Autodesk Inventor part; units mm, degrees
ref_plane "YZ Plane" through (0, 0, 0) normal (1, 0, 0) x (0, 1, 0)
ref_plane "XZ Plane" through (0, 0, 0) normal (0, 1, 0) x (-1, 0, 0)
ref_plane "XY Plane" through (0, 0, 0) normal (0, 0, 1) x (1, 0, 0)
sketch "Sketch1" plane through (0, 0, 0) normal (0, 0, 1) x (1, 0, 0)
  circle A0 centre (8.9, 50.3645) radius 1.55 construction
  circle A1 centre (8.9, 50.3645) radius 3
  circle A2 centre (51.1, 50.3645) radius 1.55 construction
  circle A3 centre (51.1, 50.3645) radius 3
  circle A4 centre (60, 0) radius 1.55
  circle A5 centre (60, 0) radius 1.55
  circle A6 centre (0, 0) radius 1.55
  circle A7 centre (0, 0) radius 1.55
  circle A8 centre (54.13, 40.8) radius 1.5999
  circle A9 centre (5.87, 42.07) radius 1.5999
  circle A10 centre (38.89, -10) radius 1.5999
  circle A11 centre (54.13, 40.8) radius 1.55 construction
  circle A12 centre (5.87, 42.07) radius 1.55 construction
  circle A13 centre (38.89, -10) radius 1.55 construction
  line L0 (8.9, 55.3645) -> (3.9, 55.3645) construction
  circle A14 centre (30, 20) radius 22.5
  arc A15 (38.89, -5) -> (37.7654, -14.8719) centre (38.89, -10) ccw construction
  arc A16 (37.6448, -14.8425) -> (41.0305, -14.5186) centre (38.89, -10) ccw
  line L1 (8.9, 55.3645) -> (8.9, 50.3645) construction
  line L2 (51.1, 55.3645) -> (51.1, 50.3645) construction
  arc A17 (-1.2452, -4.8425) -> (-5, 0) centre (0, 0) ccw construction
  arc A18 (65, 0) -> (64.9237, 0.8701) centre (60, 0) ccw
  line L3 (-1.2452, -4.8425) -> (37.6448, -14.8425)
  line L4 (41.0305, -14.5186) -> (62.1405, -4.5186)
  arc A19 (-4.9237, 0.8701) -> (-1.2452, -4.8425) centre (0, 0) ccw
  arc A20 (62.1405, -4.5186) -> (65, 0) centre (60, 0) ccw
  arc A21 (3.9763, 51.2346) -> (8.9, 55.3645) centre (8.9, 50.3645) ccw construction
  line L5 (-4.9237, 0.8701) -> (3.9763, 51.2346)
  line L6 (56.0237, 51.2346) -> (64.9237, 0.8701)
  arc A22 (64.9237, 0.8701) -> (62.1405, -4.5186) centre (60, 0) ccw construction
  arc A23 (41.0305, -14.5186) -> (38.89, -5) centre (38.89, -10) ccw construction
  line L7 (8.9, 55.3645) -> (51.1, 55.3645)
  arc A24 (8.9, 55.3645) -> (3.9763, 51.2346) centre (8.9, 50.3645) ccw
  circle A25 centre (51.1, 50.3645) radius 5
  point P0 (17, 90.5)
  dimension "d0" = 6
  dimension "d1" = 6
  dimension "d2" = 3.1
  dimension "d3" = 3.1
  dimension "d4" = 8.9
  dimension "d5" = 8.9
  dimension "d6" = 42.2
  dimension "d7" = 50.3645
  dimension "d8" = 0
  dimension "d9" = 0
  dimension "d10" = 3.1
  dimension "d11" = 3.1
  dimension "d12" = 3.1
  dimension "d13" = 52.07
  dimension "d14" = 50.8
  dimension "d15" = 33.02
  dimension "d16" = 15.24
  dimension "d19" = 5.87
  dimension "d51" = 5
  dimension "d52" = 45
  dimension "d55" = 10
  dimension "d56" = 10
  dimension "d65" = 20
  dimension "d66" = 21.1
  dimension "d67" = 10
  dimension "d68" = 10
  dimension "d69" = 10
  dimension "d71" = 10
extrude "Extrusion1" add sketch "Sketch1" along normal blind 2
sketch "Sketch5" plane through (0, 0, 2) normal (0, 0, 1) x (1, 0, 0)
  circle A0 centre (5.87, 42.07) radius 1.5999
  circle A1 centre (5.87, 42.07) radius 3
  circle A2 centre (54.13, 40.8) radius 1.5999
  circle A3 centre (54.13, 40.8) radius 3
  circle A4 centre (38.89, -10) radius 1.5999
  circle A5 centre (38.89, -10) radius 3
  point P0 (0, 0)
  dimension "d57" = 6
  dimension "d58" = 6
  dimension "d59" = 6
extrude "Extrusion5" add sketch "Sketch5" along normal blind 5
chamfer "Chamfer3" distance 1 angle 45 6 edges at (2.87, 42.07, 2) (2.87, 42.07, 7) (51.13, 40.8, 2) (51.13, 40.8, 7) (35.89, -10, 2) (35.89, -10, 7)
equation "\"d66\" = 0.5 * d6"
properties part number "SimpleRTK - PlateAdapter"
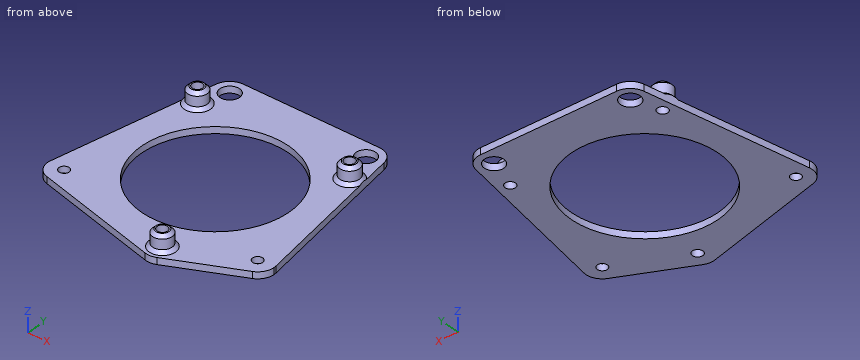
Check sheet for the modelled part. Datum: model origin and axes. Units: mm. Round coordinates to 2 decimals unless told otherwise and drop trailing zeros. Order: outer loops, then holes, each group sorted by start corner. A loop starts at its lowest first (then second) coordinate and runs counter-clockwise, first axis right, second up.
Q1. Cross-section at B-B, the plane y = 26. Enter the section's corners in (x, z), plus the area to 3 significant figures.
Filled sheet:
outline: (-0.48, 0) - (8.31, 0) - (8.31, 2) - (-0.48, 2) - close; (51.69, 0) - (60.48, 0) - (60.48, 2) - (51.69, 2) - close
area: 35.2 mm2
Q2. Cross-section at C-C, the plane x = 0. Enter the section's corners in (y, z).
Filled sheet:
outline: (-5.16, 0) - (-1.55, 0) - (-1.55, 2) - (-5.16, 2) - close; (1.55, 0) - (28.73, 0) - (28.73, 2) - (1.55, 2) - close
Q3. Scan lines: L1, parallel to Y at x = 38.89, z = 3.5; L2, parallel to X at y = 41, z = 3.5; L3, parallel to Y at x = 54.13, z = 5.5. Record each from-to range of solid material in increasing order.
Filled sheet:
L1: y = -13 to -11.6, -8.4 to -7
L2: x = 3.07 to 4.68, 7.06 to 8.67, 51.14 to 52.54, 55.72 to 57.12
L3: y = 37.8 to 39.2, 42.4 to 43.8
Q4. Cross-section at A-A, the plane z = 1. Give the number of separate pieces and of enclosed holes in the cut face, plus the area to 3 significant figures.
Filled sheet:
separate pieces: 1
enclosed holes: 8
area: 2,310 mm2
